from build123d import *

# Parameters (mm, degrees)
SKETCH1_W           = 65.5
SKETCH1_H           = 78.2
BOSS_EXTRUDE1_DEPTH = 2
SKETCH2_W           = 61.2
SKETCH2_H           = 73.9
SKETCH2_W_2         = 57.2
SKETCH2_H_2         = 69.9
BOSS_EXTRUDE2_DEPTH = 5
SKETCH3_W           = 5
SKETCH3_H           = 9.47
CUT_EXTRUDE1_DEPTH  = 2
SKETCH4_W           = 5
SKETCH4_H           = 4.9
CUT_EXTRUDE2_DEPTH  = 2
FILLET1_R           = 2
SKETCH5_W           = 25
SKETCH5_H           = 2
BOSS_EXTRUDE3_DEPTH = 8
SKETCH6_W           = 25
SKETCH6_H           = 2
BOSS_EXTRUDE4_DEPTH = 8
SKETCH7_W           = 21
SKETCH7_H           = 4
CUT_EXTRUDE3_DEPTH  = 3


with BuildPart() as part:
    # Sketch1 → Boss-Extrude1 (new body)
    with BuildSketch(Plane.XY):
        with Locations((4.011517615, -7.43604336)):
            Rectangle(SKETCH1_W, SKETCH1_H)
    extrude(amount=BOSS_EXTRUDE1_DEPTH)

    # Sketch2 → Boss-Extrude2 (add)
    with BuildSketch(Plane.XY.offset(2)):
        with Locations((4.011517615, -7.43604336)):
            Rectangle(SKETCH2_W, SKETCH2_H)
        with Locations((4.011517615, -7.43604336)):
            Rectangle(SKETCH2_W_2, SKETCH2_H_2, mode=Mode.SUBTRACT)
    extrude(amount=BOSS_EXTRUDE2_DEPTH)

    # Sketch3 → Cut-Extrude1 (cut)
    with BuildSketch(Plane(origin=(34.611517615, 0, 0), x_dir=(0, 0, -1), z_dir=(1, 0, 0))):
        with Locations((-4.5, 15.24895664)):
            Rectangle(SKETCH3_W, SKETCH3_H)
    extrude(amount=-CUT_EXTRUDE1_DEPTH, mode=Mode.SUBTRACT)

    # Sketch4 → Cut-Extrude2 (cut)
    with BuildSketch(Plane.ZY.offset(26.588482385)):
        with Locations((4.5, -7.43604336)):
            Rectangle(SKETCH4_W, SKETCH4_H)
    extrude(amount=-CUT_EXTRUDE2_DEPTH, mode=Mode.SUBTRACT)

    # Fillet1
    fillet1_edges = [part.edges().sort_by_distance(p)[0] for p in [
        (-28.738482385, 31.66395664, 1),
        (36.761517615, 31.66395664, 1),
        (36.761517615, -46.53604336, 1),
        (-28.738482385, -46.53604336, 1),
    ]]
    fillet(fillet1_edges, radius=FILLET1_R)

    # Sketch5 → Boss-Extrude3 (add)
    with BuildSketch(Plane(origin=(0, 31.66395664, 0), x_dir=(1, 0, 0), z_dir=(0, 1, 0))):
        with Locations((3.761517615, -1)):
            Rectangle(SKETCH5_W, SKETCH5_H)
    extrude(amount=BOSS_EXTRUDE3_DEPTH)

    # Sketch6 → Boss-Extrude4 (add)
    with BuildSketch(Plane.XZ.offset(46.53604336)):
        with Locations((3.761517615, 1)):
            Rectangle(SKETCH6_W, SKETCH6_H)
    extrude(amount=BOSS_EXTRUDE4_DEPTH)

    # Sketch7 → Cut-Extrude3 (cut, through all)
    with BuildSketch(Plane.XY.offset(2)):
        with Locations((3.761517615, -50.53604336)):
            Rectangle(SKETCH7_W, SKETCH7_H)
        with Locations((3.761517615, 35.66395664)):
            Rectangle(SKETCH7_W, SKETCH7_H)
    extrude(amount=-CUT_EXTRUDE3_DEPTH, mode=Mode.SUBTRACT)


solid = part.part
Could you check a few things on this model? Use its own coordinates, in mm. A direction names the side the tool comes from. Round coordinates to 2 decimals unless told otherwise and drop trailing zeros. Order: outer loops, then holes, each group sorted by start corner. A loop starts at its lowest first (then second) coordinate and runs counter-clockwise, first axis right, second up.
(1) Please list where these lines run through material, in increasing order: line 1 along Y through (x, z) = (7.5, 1.5); line 2 along X through (y, z) = (-13.5, 3.25); line 3 along Y through (x, z) = (28, 4.75).
Response values:
line 1: y = -54.54 to -52.54, -48.54 to 33.66, 37.66 to 39.66
line 2: x = -26.59 to -24.59, 32.61 to 34.61
line 3: y = -44.39 to -42.39, 27.51 to 29.51
(2) I'm going to push flat-ended pins straight in: pin 1 (2 mm diameter, centred on y = -50, z = 1, fed in from +X); pin 2 (3 mm diameter, centred on y = -30, z = 6, fed in from +X); pin 3 (1 mm diameter, centred on y = 35.5, z = 1, fed in from -X). Where does each tip first touch, or does it pass through?
Response values:
pin 1: stops at x = 16.26
pin 2: stops at x = 34.61
pin 3: stops at x = -8.74
(3) Imagine slicing it at D-D (x = 21). Write out the boundary of the cut face in (y, z), plus the area to 3 significant figures.
Response values:
outline: (-46.54, 0) - (31.66, 0) - (31.66, 2) - (29.51, 2) - (29.51, 7) - (27.51, 7) - (27.51, 2) - (-42.39, 2) - (-42.39, 7) - (-44.39, 7) - (-44.39, 2) - (-46.54, 2) - close
area: 176 mm2
(4) Imagine slicing it at C-C (y = 12.5). Write out the boundary of the cut face in (x, z), plus the area to 3 significant figures.
Response values:
outline: (-28.74, 0) - (36.76, 0) - (36.76, 2) - (-24.59, 2) - (-24.59, 7) - (-26.59, 7) - (-26.59, 2) - (-28.74, 2) - close
area: 141 mm2
(5) If we mould it in two halves opening along X, with no side actions, what happens to faces 6 (the flat face through (4, -42.386, 4)), 7 (the flat face through (-8.738, -50, 1)), 8 (the flat face through (16.262, 36, 1))? For each: released by +X, released by -X, zero draft, split by the parting line, or undercut.
Response values:
face 6: undercut
face 7: released by -X
face 8: released by +X
(6) Which directions (+Z, -Z, +X, -X, +Y, -Y) give clear straight access to the entire face, cutting with the end or side of a thin tool? Please do faces 1 (the flat face through (-18, -46.536, 1)), 2 (the flat face through (4, 29.514, 4)), 3 (the flat face through (4, -44.386, 4)), 4 (the flat face through (16.262, -50, 1)), 5 (the flat face through (14.262, 36, 1)).
Response values:
face 1: +Z, -Z, -X, -Y
face 2: +Z, +X, -X, +Y
face 3: +Z, +X, -X, -Y
face 4: +Z, -Z, +X, -Y
face 5: +Z, -Z
(7) Imagine slicing it at A-A (x = 11). Write out the boundary of the cut face in (y, z).
Response values:
outline: (-54.54, 0) - (-52.54, 0) - (-52.54, 2) - (-54.54, 2) - close; (-48.54, 0) - (33.66, 0) - (33.66, 2) - (29.51, 2) - (29.51, 7) - (27.51, 7) - (27.51, 2) - (-42.39, 2) - (-42.39, 7) - (-44.39, 7) - (-44.39, 2) - (-48.54, 2) - close; (37.66, 0) - (39.66, 0) - (39.66, 2) - (37.66, 2) - close
(8) Imagine slicing it at B-B (z = 4.75). Write out the boundary of the cut face in (x, y), plus the area to 3 significant figures.
Response values:
outline: (-26.59, -44.39) - (34.61, -44.39) - (34.61, 10.51) - (32.61, 10.51) - (32.61, -42.39) - (-24.59, -42.39) - (-24.59, -9.89) - (-26.59, -9.89) - close; (-26.59, -4.99) - (-24.59, -4.99) - (-24.59, 27.51) - (32.61, 27.51) - (32.61, 19.98) - (34.61, 19.98) - (34.61, 29.51) - (-26.59, 29.51) - close
area: 496 mm2
